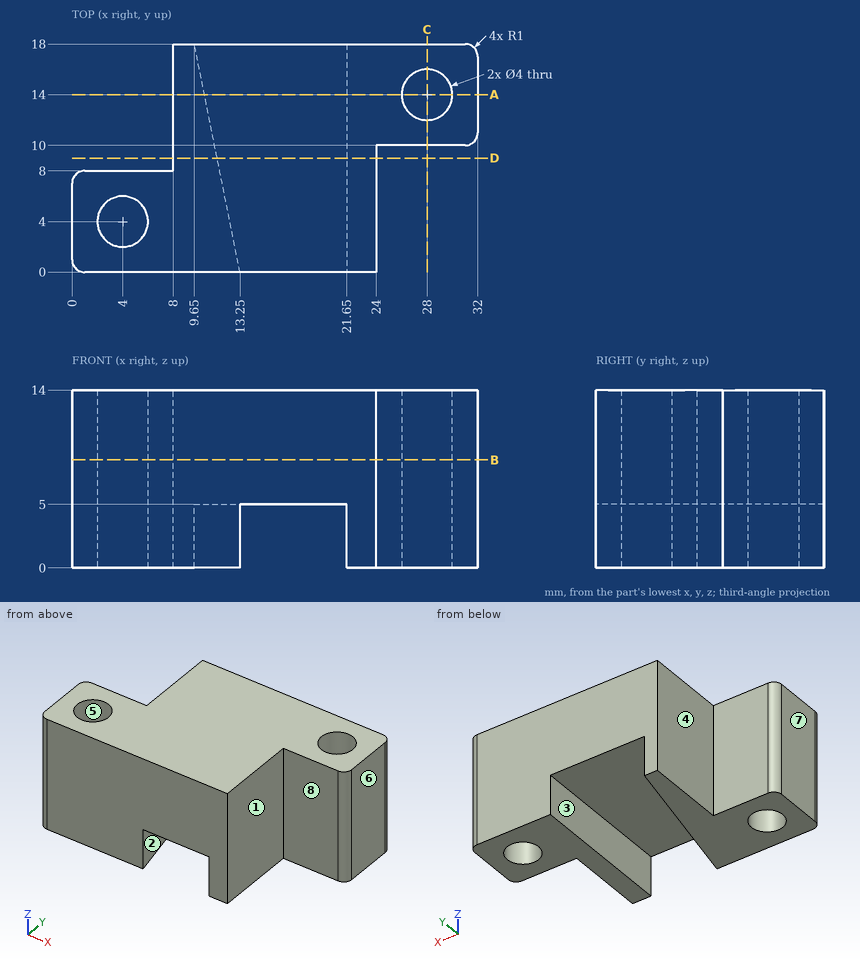
The figure shows three views and two pictorial views of one solid part (mm, origin at its lowest corner). Answer the questions. A direction names the side the tool comes from. Coordinates: 2 decimals unless noted, no trailing zeros. Loops run counter-clockwise (first coordinate to the right, second up) from the corner with the lowest first, then second, coordinate; pieces in that order, holes last. Notation, with made-up numbers: (87.5, 75.5) -> (132.5, 75.5) arc R25 ccw to (132.5, 101.5) -> close; hole circle Ø8 at (83.5, 63). An arc over 180 degrees is marked (long way). Write item = value, one per line. Start each with the question number.
1) A cutting plane is placed at C-C (x = 28). Give the vertices of the cut face in (y, z).
2) A cutting plane is placed at B-B (z = 8.5). Give the vertices of the cut face in (x, y).
3) Straight lines are drawn through the part: line 1 (Y direction, x = 28, z = 6); line 2 (Y direction, x = 4, z = 3.75); line 3 (Z direction, x = 14.5, y = 5). For each, find the intervals that lie inside material, in ascending order. Write a range as from..to.
4) Given pin 1 Ø1.5 at (y, z) = (8.5, 11) entering from -X; pin 2 Ø6 at (x, y) = (15.5, 5) entering from -Z; pin 3 Ø3 at (y, z) = (3, 8.5) entering from +X; pin 4 Ø3 at (x, y) = (4, 4) entering from -Z, each flat-ended and moving along its own axis, determine where each tip first touches the part or whether it passes through.
5) A cutting plane is placed at D-D (y = 9). Give the vertices of the cut face in (x, z), then the cut area to 3 significant figures.
6) A tool of negligible diameter and unlimited length cuts with its end or side. For the marked faces 1, 2, 3 and 4, from which of +Z, -Z, +X, -X, +Y, -Y can it reach the whole face along a straight path? Write none if from no direction.
7) The mould has two halves that part along X. Classify the marked faces 5, 6, 7 and 8: released by +X, released by -X, zero draft, split by the parting line, or undercut.
8) A cutting plane is placed at A-A (y = 14). Give the vertices of the cut face in (x, z), then the cut area to 3 significant figures.
Responses:
q1.outline = (10, 0) -> (12, 0) -> (12, 14) -> (10, 14) -> close; (16, 0) -> (18, 0) -> (18, 14) -> (16, 14) -> close
q2.outline = (0, 1) arc R1 ccw to (1, 0) -> (24, 0) -> (24, 10) -> (31, 10) arc R1 ccw to (32, 11) -> (32, 17) arc R1 ccw to (31, 18) -> (8, 18) -> (8, 8) -> (1, 8) arc R1 ccw to (0, 7) -> close; hole circle Ø4 at (4, 4); hole circle Ø4 at (28, 14)
q3.line_1 = 10..12, 16..18
q3.line_2 = 0..2, 6..8
q3.line_3 = 5..14
q4.pin_1 = 0.34
q4.pin_2 = 5
q4.pin_3 = 24
q4.pin_4 = through
q5.outline = (8, 0) -> (11.45, 0) -> (11.45, 5) -> (21.65, 5) -> (21.65, 0) -> (24, 0) -> (24, 14) -> (8, 14) -> close
q5.area = 173 mm²
q6.face_1 = +Z, -Z, +X, -Y
q6.face_2 = -Z, +Y
q6.face_3 = -Z, +Y, -Y
q6.face_4 = +Z, -Z, -X, +Y
q7.face_5 = undercut
q7.face_6 = released by +X
q7.face_7 = released by -X
q7.face_8 = zero draft
q8.outline = (8, 0) -> (10.45, 0) -> (10.45, 5) -> (21.65, 5) -> (21.65, 0) -> (26, 0) -> (26, 14) -> (8, 14) -> close; (30, 0) -> (32, 0) -> (32, 14) -> (30, 14) -> close
q8.area = 224 mm²
